```python
from build123d import *

# Parameters (mm, degrees)
F0_R     = 5
F1_DEPTH = 8
F3_DEPTH = 20
F4_R     = 7
F4_R_2   = 5
F5_DEPTH = 4
F6_DEPTH = 20.001


with BuildPart() as f1:
    # F0 (on Top) → F1 (new body)
    with BuildSketch(Plane.XY):
        with BuildLine():
            ThreePointArc((-19, 10), (-29, 0), (-19, -10))
            Line((-19, -10), (19, -10))
            ThreePointArc((19, -10), (29, 0), (19, 10))
            Line((19, 10), (-19, 10))
        make_face()
        with Locations((-19, 0)):
            Circle(F0_R, mode=Mode.SUBTRACT)
        with Locations((19, 0)):
            Circle(F0_R, mode=Mode.SUBTRACT)
    extrude(amount=F1_DEPTH)

    # F2 (on face) → F3 (join, through all)
    with BuildSketch(Plane.XZ.offset(10)):
        with BuildLine():
            Line((-10, 11), (-10, 8))
            Line((-10, 8), (0, 8))
            Line((0, 8), (10, 8))
            Line((10, 8), (10, 11))
            ThreePointArc((10, 11), (7.071068, 18.071068), (0, 21))
            ThreePointArc((0, 21), (-7.071068, 18.071068), (-10, 11))
        make_face()
    extrude(amount=-F3_DEPTH)

    # F4 (on face) → F5 (join)
    with BuildSketch(Plane.XZ.offset(10)):
        with Locations((0, 11)):
            Circle(F4_R)
        with Locations((0, 11)):
            Circle(F4_R_2, mode=Mode.SUBTRACT)
    extrude(amount=F5_DEPTH)

    # F4 (on face) → F6 (cut, through all)
    with BuildSketch(Plane.XZ.offset(10)):
        with Locations((0, 11)):
            Circle(F4_R_2)
    extrude(amount=-F6_DEPTH, mode=Mode.SUBTRACT)


solid = f1.part
```
Can you work these out from the model? Positions are in its coordinate system, mm. A direction names the side the tool comes from. Round coordinates to 2 decimals unless told otherwise and drop trailing zeros. Order: outer loops, then holes, each group sorted by start corner. A loop starts at its lowest first (then second) coordinate and runs counter-clockwise, first axis right, second up.
(1) On a 3-axis mill with a long thin cutter (end or side, diameter ignored), from which of +Z, -Z, +X, -X, +Y, -Y can I reach the whole of each face in a straight line? I mean faces 5 (the face through (29, 0, 4)), 6 (the face through (21, 5, 8)), 7 (the face through (-13, 0, 8)), 8 (the face through (0, -10, 3)), 9 (the face through (-29, 0, 4)). Say none if no direction works.
Results are:
face 5: +Z, -Z, +X
face 6: +Z, +X, +Y, -Y
face 7: +Z, -X, +Y, -Y
face 8: -Y
face 9: +Z, -Z, -X
(2) If we section it at D-D (x = 12): Please give me the cut outline in (y, z), plus the area to 3 significant figures.
Results are:
outline: (-10, 0) - (10, 0) - (10, 8) - (-10, 8) - close
area: 160 mm2
(3) If we section it at C-C (z = 17): Please give me the cut outline in (x, y).
Results are:
outline: (-8, -10) - (-3.61, -10) - (-3.61, -14) - (3.61, -14) - (3.61, -10) - (8, -10) - (8, 10) - (-8, 10) - close
(4) I'm going to push flat-ended pins straight in: pin 1 (12 mm diameter, centred on y = 5.5, z = 18, fed in from +X); pin 2 (13 mm diameter, centred on x = -19, y = 0, fed in from +Z); pin 3 (5 mm diameter, centred on x = 4, y = 1, fed in from +Z). Where does each tip first touch, or does it pass through?
Results are:
pin 1: stops at x = 9.95
pin 2: stops at z = 8
pin 3: stops at z = 20.89
(5) We'd pull the mould along X, two halves only. Please class faces 1 (the face through (0.3, 10, 5.7)), 2 (the face through (14, 0, 4)), 3 (the face through (10, 0, 9)), 4 (the face through (-1.517, -11.972, 4.166)): +X half, -X half, draft (parallel to the pull), parting line (faces both ways), or undercut.
Results are:
face 1: draft
face 2: undercut
face 3: +X half
face 4: parting line
(6) If we section it at B-B (y = -8.25): Please give me the cut outline in (x, z).
Results are:
outline: (-24.65, 0) - (24.65, 0) - (24.65, 8) - (10, 8) - (10, 11) arc R10 ccw to (0, 21) arc R10 ccw to (-10, 11) - (-10, 8) - (-24.65, 8) - close; hole circle Ø10 at (0, 11)
(7) If I drill on L1, parallel to Y at x = -19, z = 2.25; L2, parallel to Z at x = 0, y = -12.75; L3, parallel to Z at x = -16.5, y = -5.5, over which ranges is the centre line in solid material (lowest first)?
Results are:
L1: y = -10 to -5, 5 to 10
L2: z = 4 to 6, 16 to 18
L3: z = 0 to 8
(8) If we section it at A-A (y = 0): Please give me the cut outline in (x, z), plus the area to 3 significant figures.
Results are:
outline: (-29, 0) - (-24, 0) - (-24, 8) - (-29, 8) - close; (-14, 0) - (14, 0) - (14, 8) - (10, 8) - (10, 11) arc R10 ccw to (0, 21) arc R10 ccw to (-10, 11) - (-10, 8) - (-14, 8) - close; (24, 0) - (29, 0) - (29, 8) - (24, 8) - close; hole circle Ø10 at (0, 11)
area: 443 mm2
